```python
from build123d import *

# Parameters (mm, degrees)
HEX_2_DEPTH     = 3.5
THDSCHPAT_COUNT = 30
THDSCHPAT_PITCH = 0.988960665


with BuildPart() as part:
    # BodySke → BaseBody (revolve)
    with BuildSketch(Plane.XY):
        Polygon((0, 0), (0, 2.4455), (0.320140724, 3), (29, 3), (30, 2), (30, 0), align=None)
    revolve(axis=Axis((-12.7, 0, 0), (1, 0, 0)))

    # Sketch2 → Hex 2 (cut)
    with BuildSketch(Plane.ZY):
        Polygon((0.866025404, 1.5), (-0.866025404, 1.5), (-1.732050808, 0), (-0.866025404, -1.5), (0.866025404, -1.5), (1.732050808, 0), align=None)
    extrude(amount=-HEX_2_DEPTH, mode=Mode.SUBTRACT)

    # ThdSchSke → ThreadSchematic (revolve, cut)
    with BuildSketch(Plane.XY):
        Polygon((0.320140724, -2.4455), (-0.068124356, -3), (-0.068124356, -3.75), (0.708405804, -3.75), (0.708405804, -3), align=None)
    threadschematic = revolve(axis=Axis((-3.175, 0, 0), (1, 0, 0)), mode=Mode.SUBTRACT)

    # ThdSchPat: ThreadSchematic ×30
    with Locations(*[(i * THDSCHPAT_PITCH, 0, 0) for i in range(1, THDSCHPAT_COUNT)]):
        add(threadschematic, mode=Mode.SUBTRACT)


solid = part.part
```
Model file for the job. Use its own axes, mm. Give positions to 0.01 mm unless a question says otherwise; leave off trailing zeros. Use one line per item in the form item = value.
Item 1: Flat gauge pins, fed straight in: pin 1 Ø0.5 at (x, z) = (1.5, -0.5) entering from -Y; pin 2 Ø1.5 at (y, z) = (0.5, -0.5) entering from -X. Where does each tip first touch, or does it go through?
Filled in:
pin_1 = -2.98
pin_2 = 3.5
Item 2: Two-plate mould, pull along Y, no slides. Class faces 1 (the flat face through (30, 0, 0)), 2 (the flat face through (1.726, 0.74, 1.305)): released by +Y, released by -Y, zero draft, split by the parting line, or undercut.
Filled in:
face_1 = zero draft
face_2 = undercut
Item 3: Drill centre lines: L1, parallel to X at y = 1.3, z = 0.5; L2, parallel to Z at x = 2.5, y = -0.9; L3, parallel to Y at x = 19, z = 0.9. Where is each one in solid material? Low to high.
Filled in:
L1 = 3.5 to 30
L2 = -2.58 to -1.21, 1.21 to 2.58
L3 = -2.44 to 2.44
